Geometry check sheet. Reference: drawing and pictorial views, mm from the part's lowest x, y, z. Round coordinates to 2 decimals unless told otherwise and drop trailing zeros. Order: outer loops, then holes, each group sorted by start corner. A loop starts at its lowest first (then second) coordinate and runs counter-clockwise, first axis right, second up.
Q1. Cross-section at B-B on y = 2.75. Record the cut outline in (x, z), then the cut area to 3 significant figures.
Q2. Cross-section at A-A on z = 0.75. Record the cut outline in (x, y).
Q3. Scan lines: probe 1 along X at (y, z) = (9, 7.25); probe 2 along X at (y, z) = (11.5, 9); probe 3 along Y at (x, z) = (44.5, 6.75). Record each from-to range of solid material in increasing order.
Q4. Depth check by flat-ended pin: P1, Ø5, axis at y = 15, z = 4, coming from the -X side. Enter the tip coordinate at first touch or a pass-through.
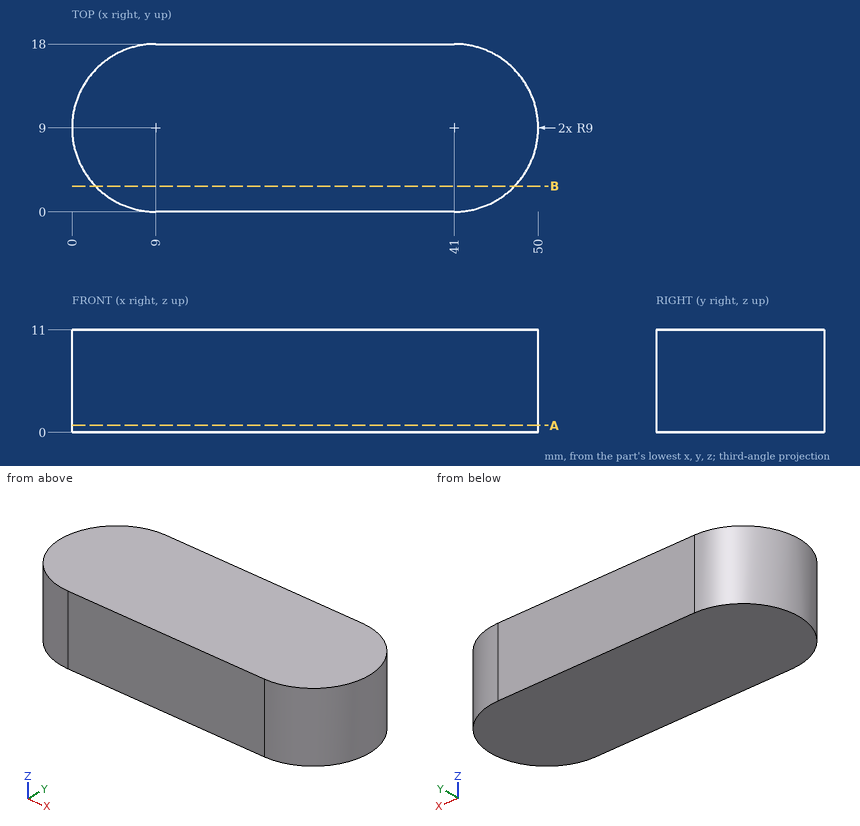
Results found:
1. outline: (2.52, 0) - (47.48, 0) - (47.48, 11) - (2.52, 11) - close
1. area: 494 mm2
2. outline: (9, 0) - (41, 0) arc R9 ccw to (41, 18) - (9, 18) arc R9 ccw to start
3. probe 1: x = 0 to 50
3. probe 2: x = 0.35 to 49.65
3. probe 3: y = 0.71 to 17.29
4. P1: stops at x = 0.71
